CAD build for the part. Positions are in the model's coordinates, mm. A direction names the side the tool comes from. Round coordinates to 2 decimals unless told otherwise and drop trailing zeros. Order: outer loops, then holes, each group sorted by start corner. A loop starts at its lowest first (then second) coordinate and runs counter-clockwise, first axis right, second up. Notation, with made-up numbers: M 12.5,67.5 L 41.5,67.5 A17 cw 41.5,80.5 Z; hole C -24,-10 d9. An arc over 180 degrees is marked long. Answer as a JSON object with one key per item and string values.
Autodesk Inventor part; units mm, degrees
ref_plane "作業平面1" through (15, 0, 0) normal (1, 0, 0) x (0, 1, 0)
ref_plane "作業平面2" through (-15, 0, 0) normal (1, 0, 0) x (0, 1, 0)
ref_plane "作業平面3" through (0, 15, 0) normal (0, 1, 0) x (-1, 0, 0)
sketch "スケッチ2" plane through (0, 0, 0) normal (0, 0, 1) x (1, 0, 0)
  circle A0 centre (0, 0) radius 15.8
  dimension "d0" = 31.6
extrude "押し出し1" add sketch "スケッチ2" against normal blind 1
sketch "スケッチ11" plane through (0, 0, -1) normal (0, 0, -1) x (-1, 0, 0)
  circle A0 centre (0, 0) radius 6
  dimension "d85" = 12
extrude "押し出し9" add sketch "スケッチ11" along normal blind 30
sketch "スケッチ12" plane through (0, 0, -31) normal (0, 0, -1) x (-1, 0, 0)
  circle A0 centre (0, 0) radius 14.8
  dimension "d106" = 29.6
extrude "押し出し10" add sketch "スケッチ12" along normal blind 10
sketch "スケッチ13" plane through (0, 0, 0) normal (0, 0, 1) x (1, 0, 0)
  circle A0 centre (0, -3) radius 1.7
  circle A1 centre (-10, -6) radius 1.7
  circle A2 centre (10, -6) radius 1.7
  line L0 (0, 0) -> (0, 17.9574) construction
  dimension "d90" = 3.4
  dimension "d91" = 3.4
  dimension "d92" = 3.4
  dimension "d93" = 3
  dimension "d94" = 6
  dimension "d95" = 10
extrude "押し出し11" cut sketch "スケッチ13" against normal through all
sketch "スケッチ14" plane through (0, 0, 0) normal (0, 0, 1) x (1, 0, 0)
  circle A0 centre (0, -11.5) radius 2.15
  circle A1 centre (9.9593, 5.75) radius 2.15
  circle A2 centre (-9.9593, 5.75) radius 2.15
  point P0 (0, 0)
  dimension "d98" = 4.3
  dimension "d99" = 11.5
  dimension "d102" = 360
extrude "押し出し12" cut sketch "スケッチ14" against normal blind 1
ref_plane "作業平面1" through (15, 0, 0) normal (1, 0, 0) x (0, 1, 0)
ref_plane "作業平面2" through (-15, 0, 0) normal (1, 0, 0) x (0, 1, 0)
ref_plane "作業平面3" through (0, 15, 0) normal (0, 1, 0) x (-1, 0, 0)
ref_plane "作業平面4" through (0, -15, 0) normal (0, 1, 0) x (-1, 0, 0)
sketch "スケッチ16" plane through (15, 0, 0) normal (1, 0, 0) x (0, 1, 0)
  circle A0 centre (0, -36) radius 1
  line L0 (-14.8, -41) -> (14.8, -41)
  point P0 (0, 0)
  dimension "d111" = 2
  dimension "d112" = 5
sketch "スケッチ17" plane through (0, 15, 0) normal (0, 1, 0) x (-1, 0, 0)
  circle A0 centre (0, -36) radius 1
  line L0 (-14.8, -41) -> (14.8, -41)
  point P0 (0, 0)
  dimension "d113" = 2
  dimension "d114" = 5
sketch "スケッチ18" plane through (-15, 0, 0) normal (1, 0, 0) x (0, 1, 0)
  circle A0 centre (0, -36) radius 1
  line L0 (-14.8, -41) -> (14.8, -41)
  point P0 (0, 0)
  dimension "d115" = 2
  dimension "d116" = 5
sketch "スケッチ19" plane through (0, -15, 0) normal (0, 1, 0) x (-1, 0, 0)
  circle A0 centre (0, -36) radius 1
  line L0 (-14.8, -41) -> (14.8, -41)
  point P0 (0, 0)
  dimension "d117" = 2
  dimension "d118" = 5
extrude "押し出し13" cut sketch "スケッチ16" against normal blind 5
extrude "押し出し14" cut sketch "スケッチ17" against normal blind 5
extrude "押し出し15" cut sketch "スケッチ18" along normal blind 5
extrude "押し出し16" cut sketch "スケッチ19" along normal blind 5
properties part number "B_pipe_cylinder_5_1" material "ステンレス鋼 440C"
Item 1: Wall check: line 1 along Z through (x, y) = (-9, 1.5); line 2 along Z through (x, y) = (0, 12); line 3 along Y through (x, z) = (0, -32). Give the ranges that are in metal, low to high. Write a range as [from, to].
Worked answers:
{"line 1": "z = [-41, -31], [-1, 0]", "line 2": "z = [-41, -37], [-35, -31], [-1, 0]", "line 3": "y = [-14.8, -4.7], [-1.3, 14.8]"}
Item 2: Saw through at B-B on x = 0. List the corners of the cut face in (y, z).
Worked answers:
{"outline": "M -15.8,-1 L -13.65,-1 L -13.65,0 L -15.8,0 Z; M -14.8,-41 L -4.7,-41 L -4.7,0 L -9.35,0 L -9.35,-1 L -6,-1 L -6,-31 L -14.8,-31 L -14.8,-35 L -10,-35 L -10,-37 L -14.8,-37 Z; M -1.3,-41 L 14.8,-41 L 14.8,-37 L 10,-37 L 10,-35 L 14.8,-35 L 14.8,-31 L 6,-31 L 6,-1 L 15.8,-1 L 15.8,0 L -1.3,0 Z"}
Item 3: Saw through at D-D on y = 0. List the corners of the cut face in (x, z).
Worked answers:
{"outline": "M -15.8,-1 L -6,-1 L -6,-31 L -14.8,-31 L -14.8,-35 L -10,-35 L -10,-37 L -14.8,-37 L -14.8,-41 L 14.8,-41 L 14.8,-37 L 10,-37 L 10,-35 L 14.8,-35 L 14.8,-31 L 6,-31 L 6,-1 L 15.8,-1 L 15.8,0 L -15.8,0 Z"}
Item 4: Saw through at A-A on y = 14. List the corners of the cut face in (x, z), and give its area (3 significant figures).
Worked answers:
{"outline": "M -7.32,-1 L 7.32,-1 L 7.32,0 L -7.32,0 Z; M -4.8,-41 L 4.8,-41 L 4.8,-31 L -4.8,-31 Z; hole C 0,-36 d2", "area": "108 mm2"}
Item 5: Drop flat-ended pins along their axis: pin 1 Ø1.8 at (x, z) = (0, -36) entering from -Y; pin 2 Ø2.5 at (x, z) = (0, -36) entering from +Y; pin 3 Ø12 at (y, z) = (5.5, -25.5) entering from -X; pin 4 Ø3 at (x, y) = (-5, -10.5) entering from +Z. Give the stop position or say it passes through.
Worked answers:
{"pin 1": "stops at y = -10", "pin 2": "stops at y = 14.8", "pin 3": "stops at x = -14.47", "pin 4": "stops at z = 0"}
Item 6: Saw through at C-C on z = -36. List the corners of the cut face in (x, y), and give its area (3 significant figures).
Worked answers:
{"outline": "M -14.77,-1 A14.8 ccw -1,-14.77 L -1,-10 L 1,-10 L 1,-14.77 A14.8 ccw 14.77,-1 L 10,-1 L 10,1 L 14.77,1 A14.8 ccw 1,14.77 L 1,10 L -1,10 L -1,14.77 A14.8 ccw -14.77,1 L -10,1 L -10,-1 Z; hole C -10,-6 d3.4; hole C 0,-3 d3.4; hole C 10,-6 d3.4", "area": "623 mm2"}
Item 7: 3-axis set-ups, long thin cutter, end or side, ignore diameter. For faces 1 (the cylindrical face through (12, 0, -35)), 2 (the flat face through (0, 10, -36)), 3 (the cylindrical face through (-13.67, 5.67, -35.93)), 4 (the cylindrical face through (0, -12, -37)), 5 (the flat face through (-6.4, 0.2, -31)): which of +Z, -Z, +X, -X, +Y, -Y reach the whole face in a straight line?
Worked answers:
{"face 1": "+X", "face 2": "+Y", "face 3": "-Z", "face 4": "-Y", "face 5": "none"}
Item 8: Two-plate mould, pull along X, no slides. Class faces 6 (the cylindrical face through (7.81, 5.84, -0.49)), 7 (the flat face through (0, 0, 0)), 8 (the cylindrical face through (-12.54, -9.61, -0.49)): released by +X, released by -X, zero draft, split by the parting line, or undercut.
Worked answers:
{"face 6": "undercut", "face 7": "zero draft", "face 8": "split by the parting line"}
